Geometry check sheet. Reference: drawing and pictorial views, mm from the part's lowest x, y, z. Round coordinates to 2 decimals unless told otherwise and drop trailing zeros. Write each loop counter-clockwise with the first axis right and the second up, starting at its lowest first coordinate (ties: lowest second). Pieces come first, ordered by that corner, then holes. Notation, with made-up numbers: M 76,-34.5 L 82,-34.5 A24 cw 82,3.5 Z; hole C 9,84 d4. An arc over 180 degrees is marked long. Use a Markdown table: item, result. Add a question column.
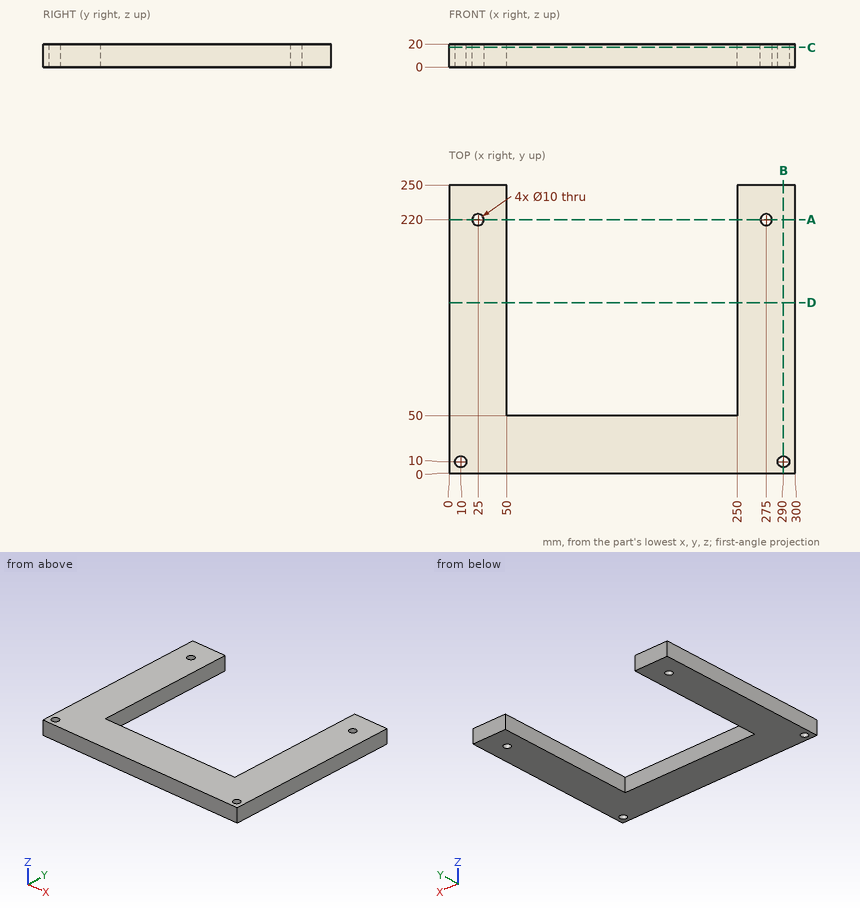
1. Scan lines: line 1 along X through (y, z) = (69.5, 2); line 2 along Y through (x, z) = (10, 13.5); line 3 along Y through (x, z) = (25, 13.25). Record each from-to range of solid material in increasing order. Write a range as from..to.
2. Depth check by flat-ended pin: pin 1 Ø8 at (x, y) = (290, 10) entering from +Z; pin 2 Ø1.5 at (x, z) = (67.5, 8.5) entering from +Y. Enter the tip coordinate at first touch or a pass-through.
3. Cross-section at A-A on y = 220. Enter the section's corners in (x, z).
4. Cross-section at B-B on x = 290. Enter the section's corners in (y, z), plus the area to 3 significant figures.
5. Cross-section at D-D on y = 148. Enter the section's corners in (x, z), plus the area to 3 significant figures.
6. Cross-section at C-C on z = 17. Enter the section's corners in (x, y), plus the area to 3 significant figures.
Answer:
| question | item | result |
|---|---|---|
| 1 | line 1 | x = 0..50, 250..300 |
| 1 | line 2 | y = 0..5, 15..250 |
| 1 | line 3 | y = 0..215, 225..250 |
| 2 | pin 1 | passes through |
| 2 | pin 2 | stops at y = 50 |
| 3 | outline | M 0,0 L 20,0 L 20,20 L 0,20 Z; M 30,0 L 50,0 L 50,20 L 30,20 Z; M 250,0 L 270,0 L 270,20 L 250,20 Z; M 280,0 L 300,0 L 300,20 L 280,20 Z |
| 4 | outline | M 0,0 L 5,0 L 5,20 L 0,20 Z; M 15,0 L 250,0 L 250,20 L 15,20 Z |
| 4 | area | 4,800 mm^2 |
| 5 | outline | M 0,0 L 50,0 L 50,20 L 0,20 Z; M 250,0 L 300,0 L 300,20 L 250,20 Z |
| 5 | area | 2,000 mm^2 |
| 6 | outline | M 0,0 L 300,0 L 300,250 L 250,250 L 250,50 L 50,50 L 50,250 L 0,250 Z; hole C 10,10 d10; hole C 25,220 d10; hole C 275,220 d10; hole C 290,10 d10 |
| 6 | area | 34,700 mm^2 |
